Here's how the part is built. I have some questions about the finished solid (model axes, mm). A direction names the side the tool comes from. Coordinates: 2 decimals unless noted, no trailing zeros. Loops run counter-clockwise (first coordinate to the right, second up) from the corner with the lowest first, then second, coordinate; pieces in that order, holes last. Notation, with made-up numbers: (21, 58) -> (31, 58) arc R21 ccw to (31, 65) -> close; hole circle Ø8 at (-12, -28). An arc over 180 degrees is marked (long way). Answer as a JSON object with one key per item and string values. Group by question number.
1) If we mould it in two halves opening along X, with no side actions, what happens to faces 6 (the flat face through (32, -0.1, -1)), 7 (the flat face through (30.5, -1, 0)), 8 (the flat face through (31.003, 52.064, 5.764))? For each: +X half, -X half, draft (parallel to the pull), parting line (faces both ways), or undercut.
2) I want a section at B-B (z = 8.5). Write out the boundary of the cut face in (x, y).
3) I'm going to push flat-ended pins straight in: pin 1 (0.5 mm diameter, centred on y = -0.5, z = 0, fed in from +X); pin 2 (1.6 mm diameter, centred on x = 0.5, z = 6, fed in from +Y); pin 3 (1.9 mm diameter, centred on x = 18.1, y = 30.76, fed in from -Z). Where does each tip first touch, or does it pass through?
4) I want a section at D-D (y = 24.5). Write out the boundary of the cut face in (x, z).
5) I want a section at C-C (x = 28.5). Write out the boundary of the cut face in (y, z).
6) I want a section at A-A (y = 17). Write out the boundary of the cut face in (x, z), then the cut area to 3 significant figures.
7) I need wall thicknesses on probe 1 along Y at (x, z) = (3.5, -0.5); probe 2 along Z at (x, y) = (14.5, 48); probe 3 along Z at (x, y) = (17, 34). Which ranges of each line are inside material? Lowest first, please. Write a range as [from, to].
8) Which directions (+Z, -Z, +X, -X, +Y, -Y) give clear straight access to the entire face, cutting with the end or side of a thin tool? Please do faces 1 (the cylindrical face through (4.032, 3.084, 5.764)), 2 (the flat face through (0, 33, 6)), 3 (the flat face through (36.3, 12, -1)), 4 (the flat face through (37, 0.06, 0)), 5 (the flat face through (36.2, 43, 1)).
```python
from build123d import *

# Parameters (mm, degrees)
DISPLAY_SUPPORT_PLATE_DEPTH           = 1.5
UNDERSIDE_LOCATING_RIM_START          = -1.3
UNDERSIDE_LOCATING_RIM_PROFILE_W      = 3.099998474
UNDERSIDE_LOCATING_RIM_PROFILE_H      = 1.499999911
UNDERSIDE_LOCATING_RIM_DEPTH          = 1.3
DISPLAY_RELIEF_PROFILE_W              = 17
DISPLAY_RELIEF_PROFILE_H              = 25
DISPLAY_RELIEF_DEPTH                  = 0.2
POSTS_AND_RETAINING_STOPS_PROFILE_R   = 2.500000022
POSTS_AND_RETAINING_STOPS_PROFILE_R_2 = 2.500000099
POSTS_AND_RETAINING_STOPS_PROFILE_W   = 2
POSTS_AND_RETAINING_STOPS_PROFILE_H   = 8.867599487
POSTS_AND_RETAINING_STOPS_DEPTH       = 8.65
LOCATING_POST_BORE_PROFILE_R          = 1.2
LOCATING_POST_BORE_DEPTH              = 8.65
BORE_ENTRY_CHAMFER_PROFILE_R          = 1.6
BORE_ENTRY_CHAMFER_DEPTH              = 0.692820323
BORE_ENTRY_CHAMFER_DRAFT              = -30


with BuildPart() as part:
    # Display_support_plate_profile → Display_support_plate (new body)
    with BuildSketch(Plane.XY):
        with BuildLine():
            Line((-0.099999994, 53.399997711), (36.200000763, 53.399997711))
            Line((36.200000763, 53.399997711), (36.200000763, 23.911094666))
            Line((36.200000763, 23.911094666), (37.799999237, 23.911094666))
            Line((37.799999237, 23.911094666), (37.799999237, 0.059999999))
            Line((37.799999237, 0.059999999), (36.200000763, 0.059999999))
            Line((36.200000763, 0.059999999), (36.200000763, 0))
            Line((36.200000763, 0), (33.599998474, 0))
            Line((33.599998474, 0), (33.599998474, -1.599999905))
            Line((33.599998474, -1.599999905), (30.5, -1.599999905))
            Line((30.5, -1.599999905), (30.5, 0))
            Line((30.5, 0), (7.699999809, 0))
            Line((7.699999809, 0), (7.699999809, -1.599999905))
            Line((7.699999809, -1.599999905), (-0.099999994, -1.599999905))
            ThreePointArc((-0.099999994, -1.599999905), (-1.160660136, -1.160660136), (-1.599999905, -0.099999994))
            Line((-1.599999905, -0.099999994), (-1.599999905, 51.899997711))
            ThreePointArc((-1.599999905, 51.899997711), (-1.160660627, 52.960658371), (-0.099999994, 53.399997711))
        make_face()
    extrude(amount=DISPLAY_SUPPORT_PLATE_DEPTH)

    # Underside_locating_rim_profile → Underside_locating_rim (add)
    with BuildSketch(Plane.XY.offset(UNDERSIDE_LOCATING_RIM_START)):
        with Locations((32.049999237, -0.84999995)):
            Rectangle(UNDERSIDE_LOCATING_RIM_PROFILE_W, UNDERSIDE_LOCATING_RIM_PROFILE_H)
        with BuildLine():
            Line((-0.099999994, -0.099999994), (7.699999809, -0.099999994))
            Line((7.699999809, -0.099999994), (7.699999809, -1.599999905))
            Line((7.699999809, -1.599999905), (-0.099999994, -1.599999905))
            ThreePointArc((-0.099999994, -1.599999905), (-1.160660103, -1.160660103), (-1.599999905, -0.099999994))
            Line((-1.599999905, -0.099999994), (-1.599999905, 4.496020254))
            Line((-1.599999905, 4.496020254), (-1.599999905, 51.899997711))
            ThreePointArc((-1.599999905, 51.899997711), (-1.160660627, 52.960658371), (-0.099999994, 53.399997711))
            Line((-0.099999994, 53.399997711), (36.200000763, 53.399997711))
            Line((36.200000763, 53.399997711), (36.200000763, 51.899997711))
            Line((36.200000763, 51.899997711), (-0.100001678, 51.899999485))
            Line((-0.100001678, 51.899999485), (-0.099999994, -0.099999994))
        make_face()
        Polygon((36.299999237, 23.911094665), (37.799999237, 23.911094665), (37.799999237, 22.93311111), (37.799999237, 0.059999999), (36.299999237, 0.059999999), align=None)
    extrude(amount=UNDERSIDE_LOCATING_RIM_DEPTH)

    # Display_relief_profile → Display_relief (cut)
    with BuildSketch(Plane.XY):
        with Locations((18.05, 25.9)):
            Rectangle(DISPLAY_RELIEF_PROFILE_W, DISPLAY_RELIEF_PROFILE_H)
    extrude(amount=DISPLAY_RELIEF_DEPTH, mode=Mode.SUBTRACT)

    # Posts_and_retaining_stops_profile → Posts_and_retaining_stops (add)
    with BuildSketch(Plane.XY.offset(1.5)):
        with Locations(Location((3.706309939, 5.563148769, 0), (0, 0, 180))):
            Circle(POSTS_AND_RETAINING_STOPS_PROFILE_R)
        with Locations(Location((25.3881588, 9.264928353, 0), (0, 0, 180))):
            Circle(POSTS_AND_RETAINING_STOPS_PROFILE_R_2)
        with Locations((1, 33.121494294)):
            Rectangle(POSTS_AND_RETAINING_STOPS_PROFILE_W, POSTS_AND_RETAINING_STOPS_PROFILE_H)
        with BuildLine():
            Line((21.687360763, 36.601463318), (21.626880424, 36.552923367))
            Line((21.626880424, 36.552923367), (21.602294922, 36.533191681))
            ThreePointArc((21.602294922, 36.533191681), (20.794438476, 35.265124808), (20.860019559, 33.763018036))
            ThreePointArc((20.860019559, 33.763018036), (25.609375503, 33.918488596), (21.687360763, 36.601463318))
        make_face()
        with BuildLine():
            Line((17.003135681, 32.186939239), (17.021439612, 32.20036124))
            Line((17.021439612, 32.20036124), (17.066467285, 32.233379364))
            ThreePointArc((17.066467285, 32.233379364), (19.77657842, 30.106586026), (16.341625109, 30.369355924))
            ThreePointArc((16.341625109, 30.369355924), (16.40750088, 31.374550646), (17.003135681, 32.186939239))
        make_face()
        with BuildLine():
            Line((9.829716682, 30.064435959), (9.817612885, 30.003588118))
            Line((9.817612885, 30.003588118), (9.812692642, 29.978853226))
            ThreePointArc((9.812692642, 29.978853226), (10.74475441, 27.921723152), (12.999830034, 28.044837762))
            ThreePointArc((12.999830034, 28.044837762), (12.856910571, 31.318323984), (9.829716682, 30.064435959))
        make_face()
        Polygon((36.200000763, 49.774204254), (36.200000763, 53.399997711), (32.290077446, 53.399997711), (30.700677872, 53.399997711), (31.313196182, 50.690540314), align=None)
    extrude(amount=POSTS_AND_RETAINING_STOPS_DEPTH)

    # Locating_post_bore_profile → Locating_post_bore (cut)
    with BuildSketch(Plane.XY.offset(10.15)):
        with Locations((18.098906, 30.758906)):
            Circle(LOCATING_POST_BORE_PROFILE_R)
    extrude(amount=-LOCATING_POST_BORE_DEPTH, mode=Mode.SUBTRACT)


with BuildPart() as bore_entry_chamfer_tool:
    # Bore_entry_chamfer_profile → Bore_entry_chamfer (with draft: the straight prism first)
    with BuildSketch(Plane.XY.offset(10.15)):
        with Locations((18.098906, 30.758906)):
            Circle(BORE_ENTRY_CHAMFER_PROFILE_R)
    extrude(amount=-BORE_ENTRY_CHAMFER_DEPTH)
    # Bore_entry_chamfer: the draft: its side faces are tilted about the plane it starts from
    bore_entry_chamfer_sides = [bore_entry_chamfer_tool.faces().sort_by_distance(p)[0] for p in [
        (16.498906, 30.758906, 9.803589838),
    ]]
    draft(bore_entry_chamfer_sides, Plane.XY.offset(10.15), BORE_ENTRY_CHAMFER_DRAFT)


with BuildPart() as part_1:
    add(part.part)

    # Bore_entry_chamfer: cut by bore_entry_chamfer_tool
    add(bore_entry_chamfer_tool.part, mode=Mode.SUBTRACT)


solid = part_1.part
```
Determined:
{
 "1": {"face 6": "draft", "face 7": "undercut", "face 8": "-X half"},
 "2": {"outline": "(0, 28.69) -> (2, 28.69) -> (2, 37.56) -> (0, 37.56) -> close; circle Ø5 at (3.71, 5.56); (9.81, 29.98) arc R2 ccw (long way) to (9.83, 30.06) -> close; (17, 32.19) arc R1.8 ccw (long way) to (17.07, 32.23) -> close; (21.6, 36.53) arc R2.5 ccw (long way) to (21.69, 36.6) -> close; circle Ø5 at (25.39, 9.26); (30.7, 53.4) -> (31.31, 50.69) -> (36.2, 49.77) -> (36.2, 53.4) -> close; hole circle Ø2.4 at (18.1, 30.76)"},
 "3": {"pin 1": "x = 33.6", "pin 2": "y = 37.56", "pin 3": "z = 0.2"},
 "4": {"outline": "(-1.6, -1.3) -> (-0.1, -1.3) -> (-0.1, 0) -> (9.55, 0) -> (9.55, 0.2) -> (26.55, 0.2) -> (26.55, 0) -> (36.2, 0) -> (36.2, 1.5) -> (-1.6, 1.5) -> close"},
 "5": {"outline": "(0, 0) -> (51.9, 0) -> (51.9, -1.3) -> (53.4, -1.3) -> (53.4, 1.5) -> (0, 1.5) -> close"},
 "6": {"outline": "(-1.6, -1.3) -> (-0.1, -1.3) -> (-0.1, 0) -> (9.55, 0) -> (9.55, 0.2) -> (26.55, 0.2) -> (26.55, 0) -> (36.3, 0) -> (36.3, -1.3) -> (37.8, -1.3) -> (37.8, 1.5) -> (-1.6, 1.5) -> close", "area": "59.6 mm^2"},
 "7": {"probe 1": "[-1.6, -0.1], [51.9, 53.4]", "probe 2": "[0, 1.5]", "probe 3": "[0.2, 1.5]"},
 "8": {"face 1": "+Z", "face 2": "+Z, -X, +Y, -Y", "face 3": "-Z, +Y, -Y", "face 4": "+Z, -Z, +X, -Y", "face 5": "+Z, -Z, +X, +Y"}
}
